from build123d import *

# Parameters (mm, degrees)
SKETCH1_R           = 26
BOSS_EXTRUDE1_DEPTH = 26
SKETCH2_R           = 23
CUT_EXTRUDE1_DEPTH  = 21
CUT_EXTRUDE2_DEPTH  = 21
SKETCH6_R           = 7
BOSS_EXTRUDE2_DEPTH = 25
CUT_EXTRUDE3_DEPTH  = 8


with BuildPart() as part:
    # Sketch1 → Boss-Extrude1 (new body)
    with BuildSketch(Plane(origin=(0, 0, 0), x_dir=(1, 0, 0), z_dir=(0, 1, 0))):
        Circle(SKETCH1_R)
    extrude(amount=BOSS_EXTRUDE1_DEPTH)

    # Sketch2 → Cut-Extrude1 (cut)
    with BuildSketch(Plane(origin=(0, 26, 0), x_dir=(1, 0, 0), z_dir=(0, 1, 0))):
        Circle(SKETCH2_R)
    extrude(amount=-CUT_EXTRUDE1_DEPTH, mode=Mode.SUBTRACT)

    # Sketch3 → Cut-Extrude2 (cut)
    with BuildSketch(Plane.XZ):
        with BuildLine():
            Line((-3.257409457, 22.262957657), (-3.50001968, 14.501403797))
            ThreePointArc((-3.50001968, 14.501403797), (-6.465637776, 8.899186938), (-12.710089015, 7.809896739))
            Line((-12.710089015, 7.809896739), (-20.166736072, 9.977612751))
            ThreePointArc((-20.166736072, 9.977612751), (-13.225168177, 18.202882373), (-3.257409457, 22.262957657))
        make_face()
        with BuildLine():
            Line((20.166736072, 9.977612751), (12.710089014, 7.809896739))
            ThreePointArc((12.710089014, 7.809896739), (6.465637775, 8.899186939), (3.50001968, 14.501403797))
            Line((3.50001968, 14.501403797), (3.257409457, 22.262957657))
            ThreePointArc((3.257409457, 22.262957657), (13.225168177, 18.202882373), (20.166736072, 9.977612751))
        make_face()
        with BuildLine():
            Line((15.721137791, -16.09645385), (11.355286691, -9.674622163))
            ThreePointArc((11.355286691, -9.674622163), (10.46162168, -3.399186938), (14.873220138, 1.152463692))
            Line((14.873220138, 1.152463692), (22.179925831, 3.781651771))
            ThreePointArc((22.179925831, 3.781651771), (21.398771617, -6.952882373), (15.721137791, -16.09645385))
        make_face()
        with BuildLine():
            Line((-10.450538575, -19.925768329), (-5.692135888, -13.789142064))
            ThreePointArc((-5.692135888, -13.789142064), (0, -11), (5.692135888, -13.789142064))
            Line((5.692135888, -13.789142064), (10.450538575, -19.925768329))
            ThreePointArc((10.450538575, -19.925768329), (0, -22.5), (-10.450538575, -19.925768329))
        make_face()
        with BuildLine():
            Line((-22.179925831, 3.781651771), (-14.873220138, 1.152463692))
            ThreePointArc((-14.873220138, 1.152463692), (-10.46162168, -3.399186938), (-11.355286691, -9.674622163))
            Line((-11.355286691, -9.674622163), (-15.721137791, -16.09645385))
            ThreePointArc((-15.721137791, -16.09645385), (-21.398771617, -6.952882373), (-22.179925831, 3.781651771))
        make_face()
    extrude(amount=-CUT_EXTRUDE2_DEPTH, mode=Mode.SUBTRACT)

    # Sketch5 → Cut-Revolve1 (revolve, cut)
    with BuildSketch(Plane.XY):
        with BuildLine():
            Line((18.5, 0), (22.5, 0))
            Line((22.5, 0), (22.5, 4))
            ThreePointArc((22.5, 4), (21.328427125, 1.171572875), (18.5, 0))
        make_face()
        Polygon((0, 0), (0, 2.5), (5, 2.5), (5, 4), (7.5, 4), (9, 0), align=None)
    revolve(axis=Axis((0, 26, 0), (0, -1, 0)), mode=Mode.SUBTRACT)

    # Sketch6 → Boss-Extrude2 (add)
    with BuildSketch(Plane(origin=(0, 5, 0), x_dir=(1, 0, 0), z_dir=(0, 1, 0))):
        Circle(SKETCH6_R)
    extrude(amount=BOSS_EXTRUDE2_DEPTH)

    # Sketch7 → Cut-Extrude3 (cut)
    with BuildSketch(Plane(origin=(0, 30, 0), x_dir=(1, 0, 0), z_dir=(0, 1, 0))):
        with BuildLine():
            Line((-1.875, 0), (-1.875, 1.942775077))
            ThreePointArc((-1.875, 1.942775077), (0, 2.7), (1.875, 1.942775077))
            Line((1.875, 1.942775077), (1.875, 0))
            Line((1.875, 0), (1.875, -1.942775077))
            ThreePointArc((1.875, -1.942775077), (0, -2.7), (-1.875, -1.942775077))
            Line((-1.875, -1.942775077), (-1.875, 0))
        make_face()
    extrude(amount=-CUT_EXTRUDE3_DEPTH, mode=Mode.SUBTRACT)


solid = part.part
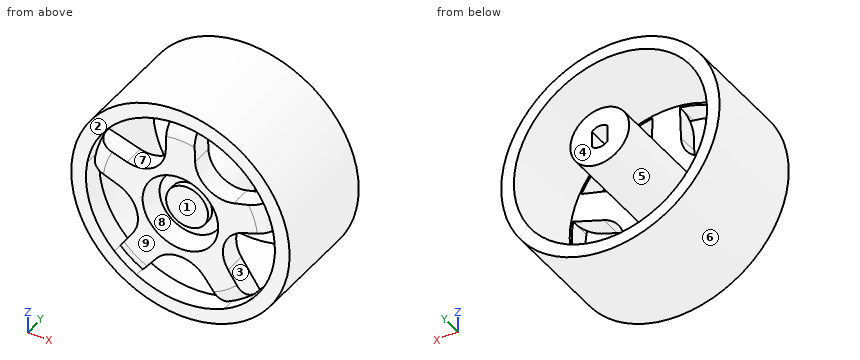
The listing builds one solid part. Answer for the finished solid, in the listing's coordinates (mm). Face numbers are marked on the shaded views. A direction names the side the tool comes from. Give positions to 0.01 mm unless a question says otherwise; leave off trailing zeros. Loops run counter-clockwise (first coordinate to the right, second up) from the corner with the lowest first, then second, coordinate; pieces in that order, holes last.
Item 1: A tool of negligible diameter and unlimited length cuts with its end or side. For the marked faces 1, 2, 3, 4 and 5, from which of +Z, -Z, +X, -X, +Y, -Y can it reach the whole face along a straight path? Write none if from no direction.
Derived:
face 1: -Y
face 2: +Z, -Z, +X, -X, -Y
face 3: +Y, -Y
face 4: +Z, -Z, +X, -X, +Y
face 5: +Y
Item 2: Determine the mould class of the marked faces 6, 7, 8 and 9 for opening direction Z: +Z half, -Z half, draft (parallel to the pull), parting line (faces both ways), or undercut.
Derived:
face 6: parting line
face 7: undercut
face 8: undercut
face 9: draft
Item 3: Find the intervals of material crossed by line 1 along Z through (x, y) = (0, 14); line 2 along X through (y, z) = (9, 4.5), in increasing order.
Derived:
line 1: z = -26 to -23, -7 to 7, 23 to 26
line 2: x = -25.61 to -22.56, -5.36 to 5.36, 22.56 to 25.61
Item 4: A cutting plane is placed at A-A (y = 18). Give the vertices of the cut face in (x, z), then the cut area to 3 significant figures.
Derived:
outline: circle Ø52 at (0, 0); circle Ø14 at (0, 0); hole circle Ø46 at (0, 0)
area: 616 mm2
Item 5: A cutting plane is placed at C-C (z = 0). Give the number of separate pieces and of enclosed holes in the cut face, then the cut area to 3 significant figures.
Derived:
separate pieces: 3
enclosed holes: 0
area: 558 mm2
Item 6: Each of these flat-tipped pins is pushed along its axis until it touches: pin 1 Ø5 at (x, y) = (-6.5, 5) entering from +Z; pin 2 Ø12 at (y, z) = (9, 15.5) entering from +X; pin 3 Ø1.5 at (x, y) = (-1, 26.5) entering from +Z. Where does it stop, or does it pass through?
Derived:
pin 1: stops at z = 25.69
pin 2: stops at x = 24.2
pin 3: stops at z = 26
